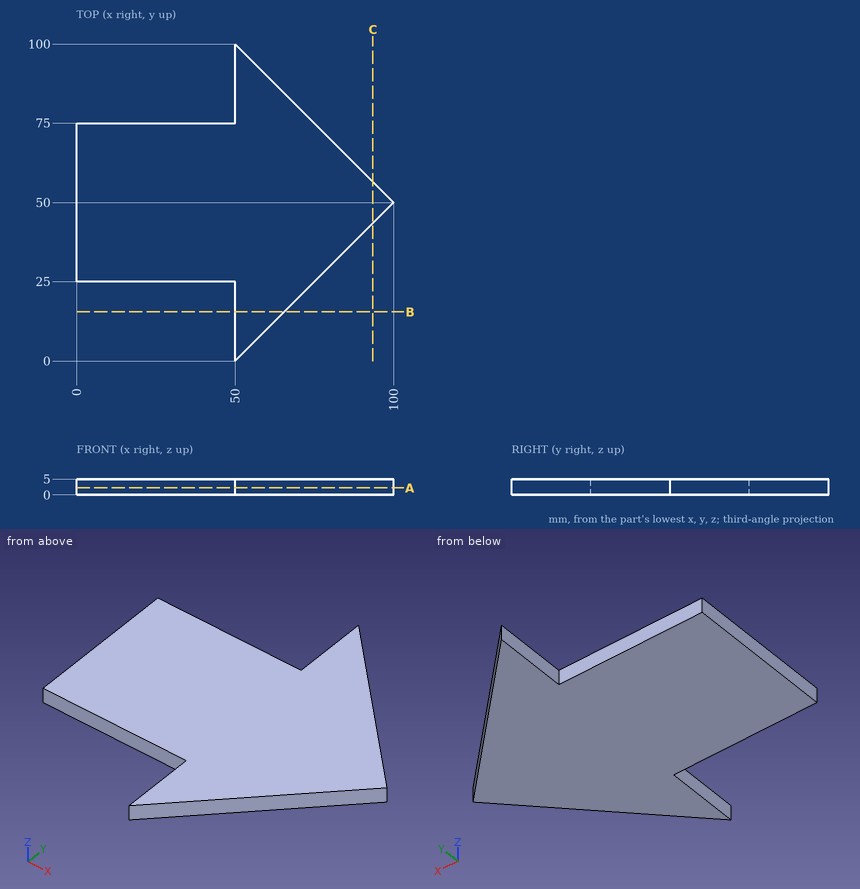
Print and shaded views of the part. All mm, measured from the part's lowest x, y and z. Give positions to 0.01 mm unless a question says otherwise; leave off trailing zeros. Order: outer loops, then holes, each group sorted by start corner. A loop starts at its lowest first (then second) coordinate and runs counter-clockwise, first axis right, second up. Notation, with made-up numbers: (2.5, -33.75) - (14.5, -33.75) arc R28 cw to (14.5, -13.75) - close; hole circle Ø2 at (22, 85). An arc over 180 degrees is marked (long way). One line per item, written item: value.
Item 1: Wall check: line 1 (Y direction, x = 25.5, z = 2.85); line 2 (Y direction, x = 56.5, z = 0.5); line 3 (X direction, y = 69, z = 1.6). Give the ranges that are in metal, low to high.
Response values:
line 1: 25 to 75
line 2: 6.5 to 93.5
line 3: 0 to 81
Item 2: Slice it at C-C (x = 93.5). List the corners of the cut face in (y, z).
Response values:
outline: (43.5, 0) - (56.5, 0) - (56.5, 5) - (43.5, 5) - close
Item 3: Slice it at B-B (y = 15.5). List the corners of the cut face in (x, z), then the cut area to 3 significant figures.
Response values:
outline: (50, 0) - (65.5, 0) - (65.5, 5) - (50, 5) - close
area: 77.5 mm2
Item 4: Pin check, flat tips, straight feed: pin 1 Ø1 at (y, z) = (85, 4) entering from +X; pin 2 Ø1.5 at (y, z) = (84, 2) entering from -X; pin 3 Ø2.5 at (x, z) = (16, 2.5) entering from -Y. Stop position of each tip, or through.
Response values:
pin 1: x = 65.5
pin 2: x = 50
pin 3: y = 25
Item 5: Slice it at A-A (z = 2.2). List the corners of the cut face in (x, y), then the cut area to 3 significant figures.
Response values:
outline: (0, 25) - (50, 25) - (50, 0) - (100, 50) - (50, 100) - (50, 75) - (0, 75) - close
area: 5,000 mm2
